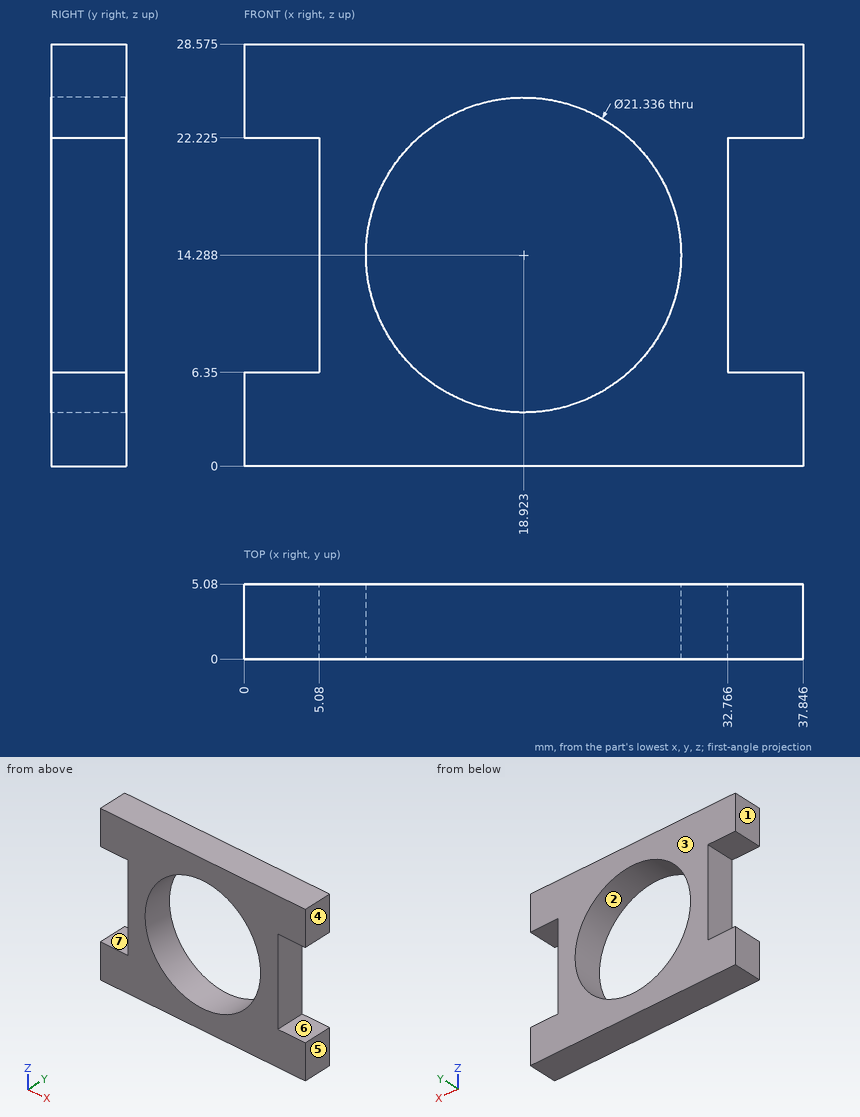
Check sheet for the drawn part. Datum: minimum x, y, z corner. Units: mm. A direction names the side the tool comes from. Give positions to 0.01 mm unless a question says otherwise; leave off trailing zeros. Write item = value, one per line. Start each with the question number.
1) Gauge pin test, flat ends, axial feed: pin 1 Ø1 at (y, z) = (4, 14.5) entering from -X; pin 2 Ø10 at (x, z) = (13.5, 13) entering from -Y; pin 3 Ø2.5 at (y, z) = (3.5, 14) entering from +X. Record the tip position at first contact, or that the pin passes through.
2) Access from +Z, -Z, +X, -X, +Y, -Y to the whole of each face (thin tool, end or side, straight path). Record for the marked faces 5, 6 and 7.
3) Scan lines: L1, parallel to Z at x = 19, y = 3.45 (1 decimal); L2, parallel to X at y = 3.45, z = 18.5 (1 decimal); L3, parallel to Z at x = 20.5, y = 1.4 (1 decimal). Record each from-to range of solid material in increasing order.
4) Draft check along X on the marked faces 1, 2, 3 and 4. Enter one of: released by +X, released by -X, zero draft, split by the parting line, or undercut.
Geometry check:
q1.pin_1 = 5.08
q1.pin_2 = through
q1.pin_3 = 32.77
q2.face_5 = +Z, -Z, +X, +Y, -Y
q2.face_6 = +X, +Y, -Y
q2.face_7 = -X, +Y, -Y
q3.L1 = 0 to 3.6, 25 to 28.6
q3.L2 = 5.1 to 9.1, 28.7 to 32.8
q3.L3 = 0 to 3.7, 24.8 to 28.6
q4.face_1 = released by -X
q4.face_2 = undercut
q4.face_3 = zero draft
q4.face_4 = released by +X
